Geometry check sheet. Reference: the model listing, model coordinates, mm. Face numbers are marked on the shaded views. Round coordinates to 2 decimals unless told otherwise and drop trailing zeros. Write each loop counter-clockwise with the first axis right and the second up, starting at its lowest first coordinate (ties: lowest second). Pieces come first, ordered by that corner, then holes. Notation, with made-up numbers: (24.5, 42.5) -> (31.5, 42.5) arc R18 ccw to (31.5, 59.5) -> close; hole circle Ø11 at (4.5, -25). An arc over 180 degrees is marked (long way). Use a Markdown table: item, result.
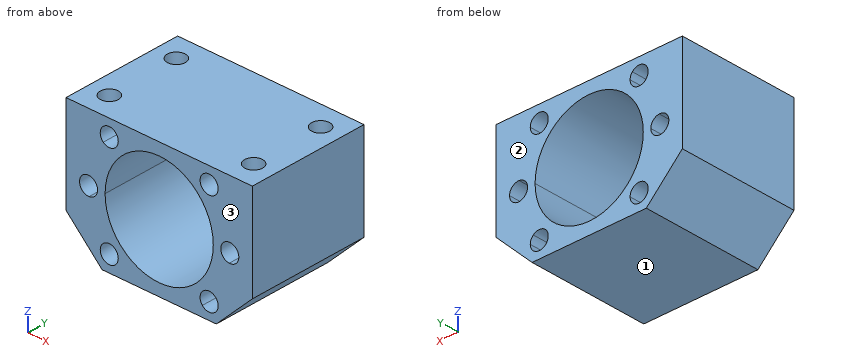
```python
from build123d import *

# Parameters (mm, degrees)
F1_DEPTH = 40
F2_R     = 3
F3_DEPTH = 16


with BuildPart() as f1:
    # F0 (on Front) → F1 (new body)
    with BuildSketch(Plane.XZ):
        with BuildLine():
            Line((0, 12), (12, 0))
            Line((12, 0), (22.738644, 0))
            ThreePointArc((22.738644, 0), (19.559896, 1.472603), (16.635389, 3.4014))
            ThreePointArc((16.635389, 3.4014), (12.26167, 3.26167), (12.4014, 7.635389))
            ThreePointArc((12.4014, 7.635389), (9.288831, 13.006939), (7.691489, 19.006118))
            ThreePointArc((7.691489, 19.006118), (4.5, 22), (7.691489, 24.993882))
            ThreePointArc((7.691489, 24.993882), (9.288831, 30.993061), (12.4014, 36.364611))
            ThreePointArc((12.4014, 36.364611), (11.38452, 38.521216), (12.26167, 40.73833))
            ThreePointArc((12.26167, 40.73833), (14.478784, 41.61548), (16.635389, 40.5986))
            ThreePointArc((16.635389, 40.5986), (19.559896, 42.527397), (22.738644, 44))
            Line((22.738644, 44), (0, 44))
            Line((0, 44), (0, 12))
        make_face()
        with BuildLine():
            ThreePointArc((12.4014, 36.364611), (9.288831, 30.993061), (7.691489, 24.993882))
            ThreePointArc((7.691489, 24.993882), (9.687975, 24.052502), (10.5, 22))
            Line((10.5, 22), (13, 22))
            ThreePointArc((13, 22), (14.370168, 28.888302), (18.272078, 34.727922))
            Line((18.272078, 34.727922), (16.504311, 36.495689))
            ThreePointArc((16.504311, 36.495689), (14.478784, 35.618539), (12.4014, 36.364611))
        make_face()
        with BuildLine():
            ThreePointArc((16.635389, 3.4014), (19.559896, 1.472603), (22.738644, 0))
            Line((22.738644, 0), (39.261356, 0))
            ThreePointArc((39.261356, 0), (42.440104, 1.472603), (45.364611, 3.4014))
            ThreePointArc((45.364611, 3.4014), (45.495689, 7.504311), (49.5986, 7.635389))
            ThreePointArc((49.5986, 7.635389), (52.711169, 13.006939), (54.308511, 19.006118))
            ThreePointArc((54.308511, 19.006118), (51.5, 22), (54.308511, 24.993882))
            ThreePointArc((54.308511, 24.993882), (52.711169, 30.993061), (49.5986, 36.364611))
            ThreePointArc((49.5986, 36.364611), (45.495689, 36.495689), (45.364611, 40.5986))
            ThreePointArc((45.364611, 40.5986), (42.440104, 42.527397), (39.261356, 44))
            Line((39.261356, 44), (22.738644, 44))
            ThreePointArc((22.738644, 44), (19.559896, 42.527397), (16.635389, 40.5986))
            ThreePointArc((16.635389, 40.5986), (17.189874, 39.675973), (17.382991, 38.617009))
            ThreePointArc((17.382991, 38.617009), (17.154629, 37.468959), (16.504311, 36.495689))
            Line((16.504311, 36.495689), (18.272078, 34.727922))
            ThreePointArc((18.272078, 34.727922), (37.888302, 38.629832), (49, 22))
            ThreePointArc((49, 22), (31, 4), (13, 22))
            Line((13, 22), (10.5, 22))
            ThreePointArc((10.5, 22), (9.687975, 19.947498), (7.691489, 19.006118))
            ThreePointArc((7.691489, 19.006118), (9.288831, 13.006939), (12.4014, 7.635389))
            ThreePointArc((12.4014, 7.635389), (15.618957, 8.116557), (17.382991, 5.382991))
            ThreePointArc((17.382991, 5.382991), (17.189874, 4.324027), (16.635389, 3.4014))
        make_face()
        with BuildLine():
            ThreePointArc((45.364611, 3.4014), (42.440104, 1.472603), (39.261356, 0))
            Line((39.261356, 0), (50, 0))
            Line((50, 0), (62, 12))
            Line((62, 12), (62, 44))
            Line((62, 44), (39.261356, 44))
            ThreePointArc((39.261356, 44), (42.440104, 42.527397), (45.364611, 40.5986))
            ThreePointArc((45.364611, 40.5986), (48.675973, 41.423893), (50.617009, 38.617009))
            ThreePointArc((50.617009, 38.617009), (50.350576, 37.381043), (49.5986, 36.364611))
            ThreePointArc((49.5986, 36.364611), (52.711169, 30.993061), (54.308511, 24.993882))
            ThreePointArc((54.308511, 24.993882), (56.552502, 24.187975), (57.5, 22))
            ThreePointArc((57.5, 22), (56.552502, 19.812025), (54.308511, 19.006118))
            ThreePointArc((54.308511, 19.006118), (52.711169, 13.006939), (49.5986, 7.635389))
            ThreePointArc((49.5986, 7.635389), (50.350576, 6.618957), (50.617009, 5.382991))
            ThreePointArc((50.617009, 5.382991), (48.675973, 2.576107), (45.364611, 3.4014))
        make_face()
    extrude(amount=F1_DEPTH)

    # F2 (on face) → F3 (cut)
    with BuildSketch(Plane.XY.offset(44)):
        with Locations((7, -8)):
            Circle(F2_R)
        with Locations((7, -32)):
            Circle(F2_R)
        with Locations((55, -32)):
            Circle(F2_R)
        with Locations((55, -8)):
            Circle(F2_R)
    extrude(amount=-F3_DEPTH, mode=Mode.SUBTRACT)


solid = f1.part
```
(1) Release check for a two-part mould opening along Y. For the marked faces 1, 2 and 3 record: +Y half, -Y half, draft (parallel to the pull), parting line (faces both ways), or undercut.
A:
| item | result |
|---|---|
| face 1 | draft |
| face 2 | +Y half |
| face 3 | -Y half |
(2) Gauge pin test, flat ends, axial feed: pin 1 Ø1.8 at (x, y) = (7.5, -7.5) entering from +Z; pin 2 Ø8 at (x, y) = (7, -32) entering from -Z; pin 3 Ø10 at (x, z) = (22.5, 19.5) entering from -Y. Record the tip position at first contact, or that the pin passes through.
A:
| item | result |
|---|---|
| pin 1 | stops at z = 28 |
| pin 2 | stops at z = 1 |
| pin 3 | passes through |
(3) Section check D-D on z = 11. Record the cut outline in (x, y), plus the area to 3 significant figures.
A:
| item | result |
|---|---|
| outline | (1, -40) -> (16.75, -40) -> (16.75, 0) -> (1, 0) -> close; (45.25, -40) -> (61, -40) -> (61, 0) -> (45.25, 0) -> close |
| area | 1,260 mm2 |
(4) Section check A-A on x = 31. Record the cut outline in (y, z).
A:
| item | result |
|---|---|
| outline | (-40, 0) -> (0, 0) -> (0, 4) -> (-40, 4) -> close; (-40, 40) -> (0, 40) -> (0, 44) -> (-40, 44) -> close |
(5) Section check B-B on z = 32.5. Record the cut outline in (x, y).
A:
| item | result |
|---|---|
| outline | (0, -40) -> (16.38, -40) -> (16.38, 0) -> (0, 0) -> close; (45.62, -40) -> (62, -40) -> (62, 0) -> (45.62, 0) -> close; hole circle Ø6 at (7, -32); hole circle Ø6 at (7, -8); hole circle Ø6 at (55, -32); hole circle Ø6 at (55, -8) |
(6) Section check C-C on y = -22.5. Record the cut outline in (x, z).
A:
| item | result |
|---|---|
| outline | (0, 12) -> (12, 0) -> (50, 0) -> (62, 12) -> (62, 44) -> (0, 44) -> close; hole circle Ø6 at (7.5, 22); hole (13, 22) arc R18 ccw (long way) to (18.27, 34.73) arc R18 ccw to start; hole (16.5, 36.5) arc R3 ccw to (17.38, 38.62) arc R3 ccw to (16.64, 40.6) arc R3 ccw (long way) to start; hole (16.64, 3.4) arc R3 ccw to (17.38, 5.38) arc R3 ccw (long way) to start; hole (49.6, 7.64) arc R3 ccw (long way) to (50.62, 5.38) arc R3 ccw to start; hole (49.6, 36.36) arc R3 ccw to (50.62, 38.62) arc R3 ccw (long way) to start; hole circle Ø6 at (54.5, 22) |
(7) Thickness scan on line 1 (Y direction, x = 7, z = 33.5); line 2 (Z direction, x = 16, y = -29.5); line 3 (Z direction, x = 7.5, y = -36.5). Record the ranges inside material, lowest first.
A:
| item | result |
|---|---|
| line 1 | y = -40 to -35, -29 to -11, -5 to 0 |
| line 2 | z = 0 to 2.86, 7.91 to 12.05, 31.95 to 36.09, 41.14 to 44 |
| line 3 | z = 4.5 to 19, 25 to 44 |
